The drawing under review shows one solid part. Ordinate dimensions are in mm from its lowest x, y, z. A direction names the side the tool comes from. Give positions to 0.01 mm unless a question says otherwise; leave off trailing zeros. Write each loop counter-clockwise with the first axis right and the second up, starting at its lowest first coordinate (ties: lowest second). Pieces come first, ordered by that corner, then holes. Notation, with made-up numbers: (59, -21) -> (88, -21) arc R30 ccw to (88, 1) -> close; hole circle Ø3 at (-26.75, -10). An arc over 180 degrees is marked (long way). Write item = value, one per line.
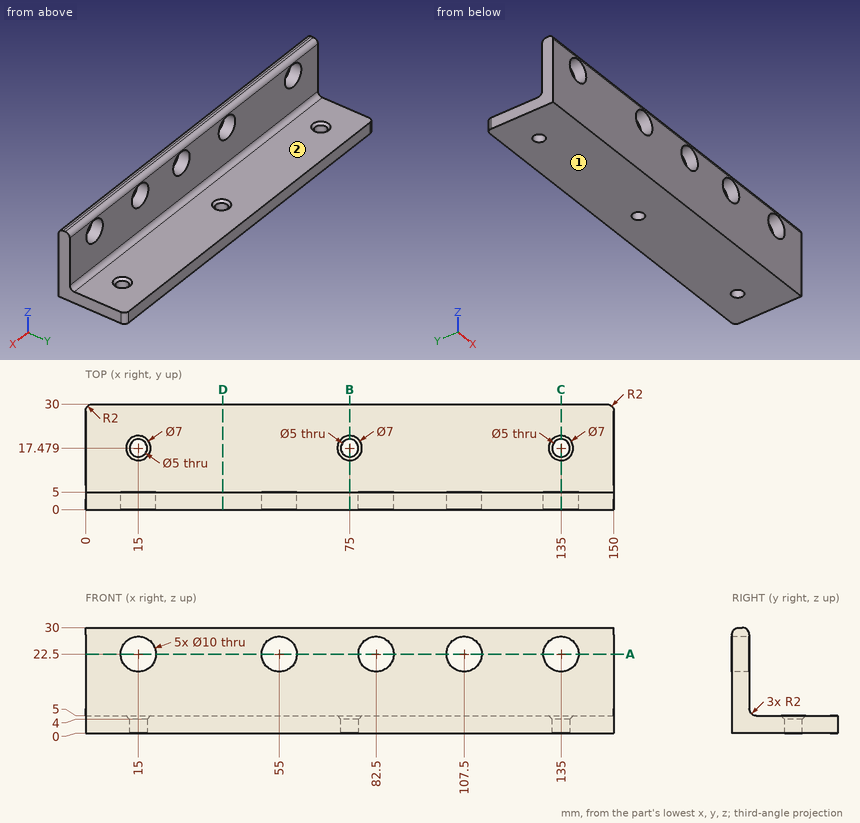
(1) To check wall thickness, follow probe 1 along X at (y, z) = (1.2, 22.5); probe 2 along Y at (x, z) = (135, 2.4); probe 3 along Z at (x, y) = (82.5, 2.4). State the ranges of each line that lie inside material, in increasing order.
Answers below:
probe_1 = 0 to 10, 20 to 50, 60 to 77.5, 87.5 to 102.5, 112.5 to 130, 140 to 150
probe_2 = 0 to 14.98, 19.98 to 30
probe_3 = 0 to 17.5, 27.5 to 30
(2) Take a section at A-A (z = 22.5). Write out the cut boundary in (x, y), plus the area to 3 significant figures.
Answers below:
outline = (0, 0) -> (10, 0) -> (10, 5) -> (0, 5) -> close; (20, 0) -> (50, 0) -> (50, 5) -> (20, 5) -> close; (60, 0) -> (77.5, 0) -> (77.5, 5) -> (60, 5) -> close; (87.5, 0) -> (102.5, 0) -> (102.5, 5) -> (87.5, 5) -> close; (112.5, 0) -> (130, 0) -> (130, 5) -> (112.5, 5) -> close; (140, 0) -> (150, 0) -> (150, 5) -> (140, 5) -> close
area = 500 mm^2
(3) Take a section at D-D (x = 39). Write out the cut boundary in (y, z).
Answers below:
outline = (0, 0) -> (30, 0) -> (30, 5) -> (7, 5) arc R2 cw to (5, 7) -> (5, 28) arc R2 ccw to (3, 30) -> (2, 30) arc R2 ccw to (0, 28) -> close
(4) Take a section at C-C (x = 135). Write out the cut boundary in (y, z), plus the area to 3 significant figures.
Answers below:
outline = (0, 0) -> (14.98, 0) -> (14.98, 4) -> (13.98, 5) -> (7, 5) arc R2 cw to (5, 7) -> (5, 17.5) -> (0, 17.5) -> close; (0, 27.5) -> (5, 27.5) -> (5, 28) arc R2 ccw to (3, 30) -> (2, 30) arc R2 ccw to (0, 28) -> close; (19.98, 0) -> (30, 0) -> (30, 5) -> (20.98, 5) -> (19.98, 4) -> close
area = 198 mm^2
(5) Take a section at B-B (x = 75). Write out the cut boundary in (y, z), plus the area to 3 significant figures.
Answers below:
outline = (0, 0) -> (14.98, 0) -> (14.98, 4) -> (13.98, 5) -> (7, 5) arc R2 cw to (5, 7) -> (5, 28) arc R2 ccw to (3, 30) -> (2, 30) arc R2 ccw to (0, 28) -> close; (19.98, 0) -> (30, 0) -> (30, 5) -> (20.98, 5) -> (19.98, 4) -> close
area = 248 mm^2
(6) For pin 1 (11.5 mm diameter, centred on x = 59.5, y = 19, fed in from +Z); pin 2 (17 mm diameter, centred on x = 107, z = 22.5, fed in from +Y); pin 3 (6 mm diameter, centred on x = 15, y = 17.48, fed in from -Z); pin 4 (6 mm diameter, centred on x = 135, y = 17.48, fed in from +Z), all flat-tipped, find the tip position at first contact; note any pin that passes through.
Answers below:
pin_1 = 5
pin_2 = 5
pin_3 = 0
pin_4 = 4.5
(7) Tool access review of the marked faces 1 and 2: name each direction out of +Z, -Z, +X, -X, +Y, -Y from which nothing blocks a thin tool from reaching the whole face with its end or side.
Answers below:
face_1 = -Z, +X, -X, +Y, -Y
face_2 = +Z, +X, -X, +Y
